Source: CAD feature listing. Evaluate the final solid. Frame: model axes, mm. A direction names the side the tool comes from. Coordinates: 2 decimals unless noted, no trailing zeros. Write each loop counter-clockwise with the first axis right and the second up, starting at its lowest first coordinate (ties: lowest second). Pieces come first, ordered by that corner, then holes. Notation, with made-up numbers: (-36, 49) -> (12, 49) arc R17 cw to (12, 69) -> close; hole circle Ø5 at (44.25, -7.75). An arc over 180 degrees is marked (long way). One line per item, written item: value. Start each with the question number.
1. Section query C-C, the plane y = 9. Output: boundary loops of the cut face in (x, z).
2. Mould query, pull axis X, two halves, no side actions, for faces 1 (the flat face through (-3, -7, -1.7)), 2 (the cylindrical face through (0.9, 9.14, 2.86)), 3 (the flat face through (-2.34, -7, 0)). Classes: released by +X, released by -X, zero draft, split by the parting line, or undercut.
3. Access query for faces 4 (the flat face through (6.5, 0, 0)), 5 (the flat face through (4, -7, -1.7)), 6 (the flat face through (-2, 5.2, 3)), 7 (the flat face through (-3, -7, 1.064)). Directions: +Z, -Z, +X, -X, +Y, -Y. A direction counts if a zero-diameter tool reaches every point of the face in a straight line with its end or side. Return the directions, or none.
4. Section query A-A, the plane x = -4.5. Output: boundary loops of the cut face in (y, z).
5. Line query: line 1 (Y direction, x = 5.75, z = 1.25); line 2 (Y direction, x = 4.75, z = 2.75); line 3 (X direction, y = 3.5, z = -2.5). Output: solid intervals per line, ascending.
6. Section query B-B, the plane y = -4.5. Output: boundary loops of the cut face in (x, z).
7. First-contact query: P1, Ø10, axis at x = 1, y = 16.5, coming from the -Z side; P2, Ø2.5, axis at x = 1, z = 1.5, coming from the -Y side; P3, Ø1, axis at y = 17, z = -1.5, coming from the -X side. Flat tips, straight axial feed; report the tip coordinate or a pass-through.
from build123d import *

# Parameters (mm, degrees)
SKETCH3_W           = 13
SKETCH3_H           = 10.4
BOSS_EXTRUDE1_DEPTH = 3.9
SKETCH4_R           = 3
BOSS_EXTRUDE2_DEPTH = 8
SKETCH6_W           = 1.669818936
SKETCH6_H           = 2.764411597
SKETCH6_W_2         = 1.648906897
BOSS_EXTRUDE3_DEPTH = 4


with BuildPart() as part:
    # Sketch3 → Boss-Extrude1 (new, symmetric)
    with BuildSketch(Plane.XY):
        Rectangle(SKETCH3_W, SKETCH3_H)
    extrude(amount=BOSS_EXTRUDE1_DEPTH, both=True)

    # Sketch4 → Boss-Extrude2 (add)
    with BuildSketch(Plane(origin=(0, 5.2, 0), x_dir=(1, 0, 0), z_dir=(0, 1, 0))):
        with Locations(Location((0, 0, 0), (0, 0, 270))):
            Circle(SKETCH4_R)
    extrude(amount=BOSS_EXTRUDE2_DEPTH)

    # Sketch5 → Revolve1 (revolve)
    with BuildSketch(Plane(origin=(-6.6, 6.6, 0), x_dir=(-0.7071067811865477, -0.7071067811865475, 0), z_dir=(0.7071067811865475, -0.7071067811865477, 0))):
        with BuildLine():
            Line((-26.301723622, 0), (-8.28734559, 0))
            add(Edge.make_bspline(
                [(-8.28734559, 0), (-9.692681087, -0.059325573), (-22.80470737, -5.257488567), (-26.301723622, 0)],
                knots=[0, 0, 0, 0, 1, 1, 1, 1], degree=3))
        make_face()
    revolve(axis=Axis((0, 13.2, 0), (0.7071067811865477, 0.7071067811865474, 0)))

    # Sketch6 → Boss-Extrude3 (add)
    with BuildSketch(Plane.XZ.offset(5.2)):
        with Locations((-3.174764559, -0.318229702)):
            Rectangle(SKETCH6_W, SKETCH6_H)
        with Locations((3.840702157, -0.318229702)):
            Rectangle(SKETCH6_W_2, SKETCH6_H)
    extrude(amount=BOSS_EXTRUDE3_DEPTH)


solid = part.part
Computed values:
1. outline: circle Ø6 at (0, 0)
2. face 1: zero draft
2. face 2: split by the parting line
2. face 3: undercut
3. face 4: +Z, -Z, +X, -Y
3. face 5: -Z, +X, -X, -Y
3. face 6: none
3. face 7: +Z, +X, -X, -Y
4. outline: (-5.2, -3.9) -> (5.2, -3.9) -> (5.2, 3.9) -> (-5.2, 3.9) -> close
5. line 1: y = -5.2 to 5.2, 16.91 to 21.72
5. line 2: y = -5.2 to 5.2
5. line 3: x = -6.5 to 6.5
6. outline: (-6.5, -3.9) -> (6.5, -3.9) -> (6.5, 3.9) -> (-6.5, 3.9) -> close
7. P1: stops at z = -3
7. P2: stops at y = -5.2
7. P3: stops at x = 2.33
